from build123d import *

# Parameters (mm, degrees)
SKETCH1_W            = 200
SKETCH1_H            = 150
BOSS_EXTRUDE1_DEPTH  = 10
SKETCH2_R            = 5
CUT_EXTRUDE1_DEPTH   = 10
SKETCH3_W            = 200
SKETCH3_H            = 150
SKETCH3_R            = 5
BOSS_EXTRUDE2_DEPTH  = 10
SKETCH4_W            = 200
SKETCH4_H            = 150
SKETCH4_R            = 5
BOSS_EXTRUDE3_DEPTH  = 10
BOSS_EXTRUDE13_START = 205
SKETCH21_R           = 5
BOSS_EXTRUDE13_DEPTH = 205
SKETCH22_R           = 5
BOSS_EXTRUDE14_DEPTH = 15
FILLET2_R            = 10
SKETCH23_R           = 1.5
CUT_EXTRUDE2_DEPTH   = 10
SKETCH30_W           = 66
SKETCH30_H           = 47
BOSS_EXTRUDE16_DEPTH = 1


with BuildPart() as part:
    # Sketch1 → Boss-Extrude1 (new body)
    with BuildSketch(Plane(origin=(0, 0, 0), x_dir=(1, 0, 0), z_dir=(0, 1, 0))):
        Rectangle(SKETCH1_W, SKETCH1_H)
    extrude(amount=BOSS_EXTRUDE1_DEPTH)

    # Sketch2 → Cut-Extrude1 (cut)
    with BuildSketch(Plane(origin=(0, 10, 0), x_dir=(1, 0, 0), z_dir=(0, 1, 0))):
        with Locations(Location((-90, 65, 0), (0, 0, 270))):
            Circle(SKETCH2_R)
        with Locations(Location((90, 65, 0), (0, 0, 90))):
            Circle(SKETCH2_R)
        with Locations(Location((90, -65, 0), (0, 0, 270))):
            Circle(SKETCH2_R)
        with Locations(Location((-90, -65, 0), (0, 0, 90))):
            Circle(SKETCH2_R)
    extrude(amount=-CUT_EXTRUDE1_DEPTH, mode=Mode.SUBTRACT)



with BuildPart() as body_2:
    # Sketch3 → Boss-Extrude2 (new body)
    with BuildSketch(Plane(origin=(0, 100, 0), x_dir=(1, 0, 0), z_dir=(0, 1, 0))):
        Rectangle(SKETCH3_W, SKETCH3_H)
        with Locations(Location((-90, 65, 0), (0, 0, 270))):
            Circle(SKETCH3_R, mode=Mode.SUBTRACT)
        with Locations(Location((90, 65, 0), (0, 0, 90))):
            Circle(SKETCH3_R, mode=Mode.SUBTRACT)
        with Locations(Location((-90, -65, 0), (0, 0, 90))):
            Circle(SKETCH3_R, mode=Mode.SUBTRACT)
        with Locations(Location((90, -65, 0), (0, 0, 270))):
            Circle(SKETCH3_R, mode=Mode.SUBTRACT)
    extrude(amount=BOSS_EXTRUDE2_DEPTH)



with BuildPart() as body_3:
    # Sketch4 → Boss-Extrude3 (new body)
    with BuildSketch(Plane(origin=(0, 200, 0), x_dir=(1, 0, 0), z_dir=(0, 1, 0))):
        Rectangle(SKETCH4_W, SKETCH4_H)
        with Locations(Location((-90, 65, 0), (0, 0, 270))):
            Circle(SKETCH4_R, mode=Mode.SUBTRACT)
        with Locations(Location((90, 65, 0), (0, 0, 90))):
            Circle(SKETCH4_R, mode=Mode.SUBTRACT)
        with Locations(Location((90, -65, 0), (0, 0, 270))):
            Circle(SKETCH4_R, mode=Mode.SUBTRACT)
        with Locations(Location((-90, -65, 0), (0, 0, 90))):
            Circle(SKETCH4_R, mode=Mode.SUBTRACT)
    extrude(amount=BOSS_EXTRUDE3_DEPTH)


with BuildPart() as body_2_1:
    add(body_2.part)

    add(body_3.part)  # Boss-Extrude13 merges body 3
    # Sketch21 → Boss-Extrude13 (add)
    with BuildSketch(Plane(origin=(0, 10, 0), x_dir=(1, 0, 0), z_dir=(0, 1, 0)).offset(BOSS_EXTRUDE13_START)):
        with Locations(Location((-90, -65, 0), (0, 0, 90))):
            Circle(SKETCH21_R)
        with Locations(Location((-90, 65, 0), (0, 0, 270))):
            Circle(SKETCH21_R)
        with Locations(Location((90, 65, 0), (0, 0, 90))):
            Circle(SKETCH21_R)
        with Locations(Location((90, -65, 0), (0, 0, 270))):
            Circle(SKETCH21_R)
    extrude(amount=-BOSS_EXTRUDE13_DEPTH)


with BuildPart() as part_1:
    add(part.part)

    add(body_2_1.part)  # Boss-Extrude14 merges body 2
    # Sketch22 → Boss-Extrude14 (add)
    with BuildSketch(Plane(origin=(0, 10, 0), x_dir=(1, 0, 0), z_dir=(0, 1, 0))):
        with Locations(Location((-90, 65, 0), (0, 0, 270))):
            Circle(SKETCH22_R)
        with Locations(Location((-90, -65, 0), (0, 0, 270))):
            Circle(SKETCH22_R)
        with Locations(Location((90, -65, 0), (0, 0, 270))):
            Circle(SKETCH22_R)
        with Locations(Location((90, 65, 0), (0, 0, 270))):
            Circle(SKETCH22_R)
    extrude(amount=-BOSS_EXTRUDE14_DEPTH)

    # Fillet2
    fillet2_edges = [part_1.edges().sort_by_distance(p)[0] for p in [
        (100, 105, 75),
        (100, 105, -75),
        (-100, 105, -75),
        (-100, 105, 75),
        (100, 205, 75),
        (100, 205, -75),
        (-100, 205, -75),
        (-100, 205, 75),
        (100, 5, 75),
        (-100, 5, 75),
        (-100, 5, -75),
        (100, 5, -75),
    ]]
    fillet(fillet2_edges, radius=FILLET2_R)

    # Sketch23 → Cut-Extrude2 (cut)
    with BuildSketch(Plane(origin=(0, 210, 0), x_dir=(1, 0, 0), z_dir=(0, 1, 0))):
        with Locations(Location((-75, 25, 0), (0, 0, 270))):
            Circle(SKETCH23_R)
        with Locations(Location((-75, -25, 0), (0, 0, 90))):
            Circle(SKETCH23_R)
        with Locations(Location((75, -25, 0), (0, 0, 270))):
            Circle(SKETCH23_R)
        with Locations(Location((75, 25, 0), (0, 0, 90))):
            Circle(SKETCH23_R)
    extrude(amount=-CUT_EXTRUDE2_DEPTH, mode=Mode.SUBTRACT)

    # Sketch30 → Boss-Extrude16 (add)
    with BuildSketch(Plane(origin=(0, 200, 0), x_dir=(-1, 0, 0), z_dir=(0, -1, 0))):
        Rectangle(SKETCH30_W, SKETCH30_H)
    extrude(amount=BOSS_EXTRUDE16_DEPTH)


solid = part_1.part
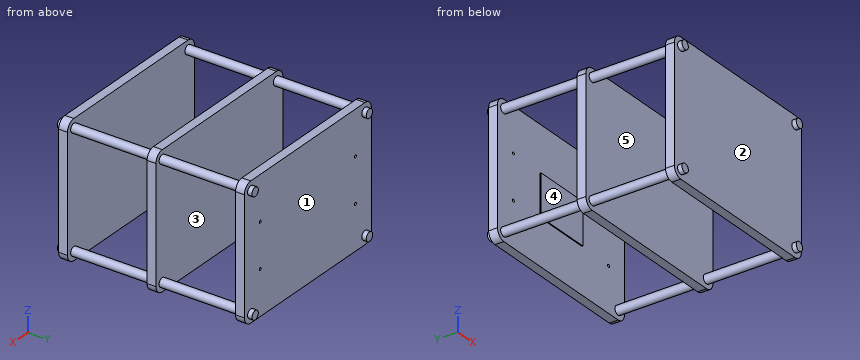
CAD build for the part. Positions are in the model's coordinates, mm. Face numbers are marked on the shaded views. A direction names the side the tool comes from. Coordinates: 2 decimals unless noted, no trailing zeros. Write each loop counter-clockwise with the first axis right and the second up, starting at its lowest first coordinate (ties: lowest second). Pieces come first, ordered by that corner, then holes. Notation, with made-up numbers: M 38,10.25 L 82,10.25 A35 cw 82,48.25 Z; hole C 38,-27 d4. An arc over 180 degrees is marked long. Answer as a JSON object with one key per item and string values. Group by question number.
1) Saw through at B-B (x = -42). Write the cut outline in (y, z).
2) Tool access for the marked faces 1, 2 and 3: list every direction of +Z, -Z, +X, -X, +Y, -Y with a clear straight run to the whole face (end or side of a thin tool).
3) Saw through at D-D (x = 1.5). Write the cut outline in (y, z).
4) Wall check: line 1 (Z direction, x = 75, y = 203.25); line 2 (Y direction, x = 41, z = 64); line 3 (X direction, y = 204, z = -25). Give the ranges that are in metal, low to high. Write a range as from..to.
5) Pin check, flat tips, straight feed: pin 1 Ø10 at (x, z) = (-30, 9.5) entering from +Y; pin 2 Ø1.8 at (x, z) = (-75, -25) entering from -Y; pin 3 Ø0.8 at (y, z) = (199.5, -7) entering from -X. Stop position of each tip, or through.
6) Saw through at A-A (z = 52). Write the cut outline in (x, y), plus the area to 3 significant figures.
7) Saw through at C-C (y = 176). Write the cut outline in (x, z).
8) Mould opens along X. For the marked faces 4 and 5 say: +X half, -X half, draft (parallel to the pull), parting line (faces both ways), or undercut.
Values follow:
{
 "1": {"outline": "M 0,-75 L 10,-75 L 10,75 L 0,75 Z; M 100,-75 L 110,-75 L 110,75 L 100,75 Z; M 200,-75 L 210,-75 L 210,75 L 200,75 Z"},
 "2": {"face 1": "+Y", "face 2": "-Y", "face 3": "none"},
 "3": {"outline": "M 0,-75 L 10,-75 L 10,75 L 0,75 Z; M 100,-75 L 110,-75 L 110,75 L 100,75 Z; M 199,-23.5 L 200,-23.5 L 200,-75 L 210,-75 L 210,75 L 200,75 L 200,23.5 L 199,23.5 Z"},
 "4": {"line 1": "z = -75..-26.5, -23.5..23.5, 26.5..75", "line 2": "y = 0..10, 100..110, 200..210", "line 3": "x = -100..-76.5, -73.5..73.5, 76.5..100"},
 "5": {"pin 1": "stops at y = 210", "pin 2": "stops at y = 0", "pin 3": "stops at x = -33"},
 "6": {"outline": "M -100,0 L 100,0 L 100,10 L -100,10 Z; M -100,100 L 100,100 L 100,110 L -100,110 Z; M -100,200 L 100,200 L 100,210 L -100,210 Z", "area": "6,000 mm2"},
 "7": {"outline": "C -90,-65 d10; C -90,65 d10; C 90,-65 d10; C 90,65 d10"},
 "8": {"face 4": "draft", "face 5": "undercut"}
}
